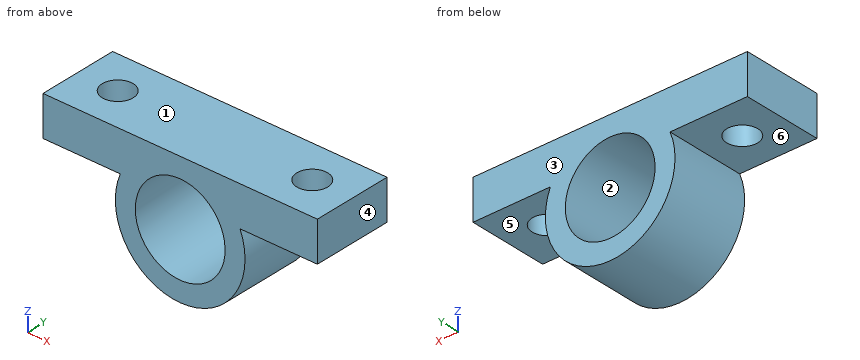
from build123d import *

# Parameters (mm, degrees)
SKETCH1_R           = 6.5
BOSS_EXTRUDE1_DEPTH = 8
SKETCH3_W           = 27.5
SKETCH3_H           = 8
BOSS_EXTRUDE2_DEPTH = 4
CUT_EXTRUDE1_REACH  = 19.185
SKETCH4_R           = 4.5
CUT_EXTRUDE2_REACH  = 20.277
SKETCH5_R           = 1.55


with BuildPart() as part:
    # Sketch1 → Boss-Extrude1 (new body)
    with BuildSketch(Plane(origin=(0, 0, 0), x_dir=(1, 0, 0), z_dir=(0, 1, 0))):
        with Locations(Location((0, 0, 0), (0, 0, 270))):
            Circle(SKETCH1_R)
    extrude(amount=BOSS_EXTRUDE1_DEPTH)

    # Sketch3 → Boss-Extrude2 (add)
    with BuildSketch(Plane(origin=(0, 8, 6.5), x_dir=(1, 0, 0), z_dir=(0, 0, 1))):
        with Locations((0, -4)):
            Rectangle(SKETCH3_W, SKETCH3_H)
    extrude(amount=-BOSS_EXTRUDE2_DEPTH)

    # Sketch4 → Cut-Extrude1 (cut, up to next)
    with BuildSketch(Plane(origin=(0, 8, 0), x_dir=(1, 0, 0), z_dir=(0, 1, 0)), mode=Mode.PRIVATE) as cut_extrude1_sk1:
        with Locations(Location((0, 0, 0), (0, 0, 270))):
            Circle(SKETCH4_R)
    cut_extrude1_tool1 = extrude(cut_extrude1_sk1.sketch, amount=-CUT_EXTRUDE1_REACH, mode=Mode.PRIVATE) & part.part
    add(cut_extrude1_tool1.solids().sort_by_distance((0, 8, 0))[0], mode=Mode.SUBTRACT)

    # Sketch5 → Cut-Extrude2 (cut, up to next)
    with BuildSketch(Plane(origin=(0, 0, 2.5), x_dir=(-1, 0, 0), z_dir=(0, 0, -1)), mode=Mode.PRIVATE) as cut_extrude2_sk1:
        with Locations((9.75, 4)):
            Circle(SKETCH5_R)
    cut_extrude2_tool1 = extrude(cut_extrude2_sk1.sketch, amount=-CUT_EXTRUDE2_REACH, mode=Mode.PRIVATE) & part.part
    # Sketch5 → Cut-Extrude2 (cut, up to next)
    with BuildSketch(Plane(origin=(0, 0, 2.5), x_dir=(-1, 0, 0), z_dir=(0, 0, -1)), mode=Mode.PRIVATE) as cut_extrude2_sk2:
        with Locations((-9.75, 4)):
            Circle(SKETCH5_R)
    cut_extrude2_tool2 = extrude(cut_extrude2_sk2.sketch, amount=-CUT_EXTRUDE2_REACH, mode=Mode.PRIVATE) & part.part
    add(cut_extrude2_tool1.solids().sort_by_distance((-9.75, 4, 2.5))[0], mode=Mode.SUBTRACT)
    add(cut_extrude2_tool2.solids().sort_by_distance((9.75, 4, 2.5))[0], mode=Mode.SUBTRACT)


solid = part.part
Work out the finished part from the listing and answer in its coordinate system (mm). Face numbers are marked on the shaded views. A direction names the side the tool comes from. Round coordinates to 2 decimals unless told otherwise and drop trailing zeros. Loops run counter-clockwise (first coordinate to the right, second up) from the corner with the lowest first, then second, coordinate; pieces in that order, holes last. Notation, with made-up numbers: (13.25, -38) - (22.25, -38) arc R19 cw to (22.25, -30) - close; hole circle Ø4 at (78, 15.5). An arc over 180 degrees is marked (long way). Use one line per item in the form item = value. Start each with the question number.
(1) Flat-ended cylindrical pins translate along their axes: P1, Ø4, axis at y = 3, z = -2, coming from the +X side; P2, Ø4, axis at x = 9.75, y = 4, coming from the -Z side; P3, Ø2, axis at y = 4.5, z = -2.5, coming from the -X side. Find the tip coordinate at first contact, or state that the pin passes through.
(2) Which of the six approach directions +Z, -Z, +X, -X, +Y, -Y give full straight-line access (tool end or side, diameter ignored) to the marked faces 4, 5 and 6?
(3) Consider line 1 (Z direction, x = -0.25, y = 3.5); line 2 (X direction, y = 4.5, z = 3.25); line 3 (Y direction, x = 10.25, z = 4). Determine where each line is inside the solid, lowest interval first.
(4) Find section A-A on x = -9.75. Determine the outline of the cut face in (y, z).
(5) Find section B-B on z = 0. Determine the outline of the cut face in (x, y).
(6) Find section D-D on y = 6. Determine the outline of the cut face in (x, z).
(7) Determine the mould class of the marked faces 1, 2 and 3 for opening direction Z: +Z half, -Z half, draft (parallel to the pull), parting line (faces both ways), or undercut.
(8) Find section C-C on y = 4.75. Determine the outline of the cut face in (x, z).
Answer list:
q1.P1 = 6.5
q1.P2 = 2.5
q1.P3 = -6.32
q2.face_4 = +Z, -Z, +X, +Y, -Y
q2.face_5 = +X, +Y, -Y
q2.face_6 = -X, +Y, -Y
q3.line_1 = -6.5 to -4.49, 4.49 to 6.5
q3.line_2 = -13.75 to -11.22, -8.28 to -3.11, 3.11 to 8.28, 11.22 to 13.75
q3.line_3 = 0 to 2.53, 5.47 to 8
q4.outline = (0, 2.5) - (2.45, 2.5) - (2.45, 6.5) - (0, 6.5) - close; (5.55, 2.5) - (8, 2.5) - (8, 6.5) - (5.55, 6.5) - close
q5.outline = (-6.5, 0) - (-4.5, 0) - (-4.5, 8) - (-6.5, 8) - close; (4.5, 0) - (6.5, 0) - (6.5, 8) - (4.5, 8) - close
q6.outline = (-13.75, 2.5) - (-6, 2.5) arc R6.5 ccw (long way) to (6, 2.5) - (13.75, 2.5) - (13.75, 6.5) - (-13.75, 6.5) - close; hole circle Ø9 at (0, 0)
q7.face_1 = +Z half
q7.face_2 = undercut
q7.face_3 = draft
q8.outline = (-13.75, 2.5) - (-11.11, 2.5) - (-11.11, 6.5) - (-13.75, 6.5) - close; (-8.39, 2.5) - (-6, 2.5) arc R6.5 ccw (long way) to (6, 2.5) - (8.39, 2.5) - (8.39, 6.5) - (-8.39, 6.5) - close; (11.11, 2.5) - (13.75, 2.5) - (13.75, 6.5) - (11.11, 6.5) - close; hole circle Ø9 at (0, 0)
